Here's how the part is built. I have some questions about the finished solid (model axes, mm). A direction names the side the tool comes from. Round coordinates to 2 decimals unless told otherwise and drop trailing zeros. Order: outer loops, then holes, each group sorted by start corner. A loop starts at its lowest first (then second) coordinate and runs counter-clockwise, first axis right, second up. Notation, with made-up numbers: (60.25, 30.5) -> (117.25, 30.5) arc R22 cw to (117.25, 60.5) -> close; hole circle Ø6 at (63.25, -15.5). An arc over 180 degrees is marked (long way). Answer in a Markdown table with one row per item.
```python
from build123d import *

# Parameters (mm, degrees)
F1_DEPTH = 82
F2_R     = 5.5
F3_DEPTH = 16.001
F4_R     = 14
F5_R     = 14


with BuildPart() as f1:
    # F0 (on Front) → F1 (new body)
    with BuildSketch(Plane.XZ):
        with BuildLine():
            Line((0, 16), (0, 0))
            Line((0, 0), (38, 0))
            Line((38, 0), (38, -4))
            Line((38, -4), (98, -4))
            Line((98, -4), (98, 0))
            Line((98, 0), (136, 0))
            Line((136, 0), (136, 16))
            Line((136, 16), (92, 16))
            ThreePointArc((92, 16), (90.070466, 13.197483), (86.763932, 14))
            Line((86.763932, 14), (49.236068, 14))
            ThreePointArc((49.236068, 14), (45.929534, 13.197483), (44, 16))
            Line((44, 16), (0, 16))
        make_face()
    extrude(amount=-F1_DEPTH)

    # F2 (on Top) → F3 (cut, through all)
    with BuildSketch(Plane.XY):
        with Locations((14, 68)):
            Circle(F2_R)
        with Locations((14, 14)):
            Circle(F2_R)
        with Locations((122, 68)):
            Circle(F2_R)
        with Locations((122, 14)):
            Circle(F2_R)
    extrude(amount=F3_DEPTH, mode=Mode.SUBTRACT)

    # F4
    f4_edges = [f1.edges().sort_by_distance(p)[0] for p in [
        (136, 0, 8),
        (136, 82, 8),
    ]]
    fillet(f4_edges, radius=F4_R)

    # F5
    f5_edges = [f1.edges().sort_by_distance(p)[0] for p in [
        (0, 0, 8),
        (0, 82, 8),
    ]]
    fillet(f5_edges, radius=F5_R)


solid = f1.part
```
1. For pin 1 Ø19 at (x, y) = (69, 23.5) entering from +Z; pin 2 Ø14.5 at (x, y) = (122, 68) entering from -Z; pin 3 Ø4.5 at (y, z) = (22, -2.5) entering from -X, each with a flat end and sliding along its axis, tell me the tip position at first contact or that it passes through.
Numbers:
| item | result |
|---|---|
| pin 1 | stops at z = 14 |
| pin 2 | stops at z = 0 |
| pin 3 | stops at x = 38 |
2. For faces 1 (the face through (98, 40, -2)), 2 (the face through (38, 40, -2)), 3 (the face through (19.08, 11.89, 7.89)), 4 (the face through (68, 40, 14)), which set-ups out of +Z, -Z, +X, -X, +Y, -Y let a thin tool reach every point of the face, with its end or its side?
Numbers:
| item | result |
|---|---|
| face 1 | -Z, +X, +Y, -Y |
| face 2 | -Z, -X, +Y, -Y |
| face 3 | +Z, -Z |
| face 4 | +Z, +Y, -Y |
3. We'd pull the mould along X, two halves only. Please class faces 5 (the face through (4, 77.8, 7.9)), 6 (the face through (131.8, 78, 8.1)), 7 (the face through (13.284, 73.453, 7.888)): released by +X, released by -X, zero draft, split by the parting line, or undercut.
Numbers:
| item | result |
|---|---|
| face 5 | released by -X |
| face 6 | released by +X |
| face 7 | undercut |
4. Suppose I cut it at D-D on x = 66. Write out the boundary of the cut face in (y, z), then the cut area to 3 significant figures.
Numbers:
| item | result |
|---|---|
| outline | (0, -4) -> (82, -4) -> (82, 14) -> (0, 14) -> close |
| area | 1,480 mm2 |
5. Suppose I cut it at C-C on x = 10. Write out the boundary of the cut face in (y, z).
Numbers:
| item | result |
|---|---|
| outline | (0.58, 0) -> (10.23, 0) -> (10.23, 16) -> (0.58, 16) -> close; (17.77, 0) -> (64.23, 0) -> (64.23, 16) -> (17.77, 16) -> close; (71.77, 0) -> (81.42, 0) -> (81.42, 16) -> (71.77, 16) -> close |
6. Please list where these lines run through material, in increasing order: line 1 along Y through (x, z) = (122, 10.75); line 2 along X through (y, z) = (14, 7.75); line 3 along Y through (x, z) = (127, 0.5).
Numbers:
| item | result |
|---|---|
| line 1 | y = 0 to 8.5, 19.5 to 62.5, 73.5 to 82 |
| line 2 | x = 0 to 8.5, 19.5 to 116.5, 127.5 to 136 |
| line 3 | y = 0.92 to 11.71, 16.29 to 65.71, 70.29 to 81.08 |
7. Suppose I cut it at A-A on y = 47. Write out the boundary of the cut face in (x, z), then the cut area to 3 significant figures.
Numbers:
| item | result |
|---|---|
| outline | (0, 0) -> (38, 0) -> (38, -4) -> (98, -4) -> (98, 0) -> (136, 0) -> (136, 16) -> (92, 16) arc R3 cw to (86.76, 14) -> (49.24, 14) arc R3 cw to (44, 16) -> (0, 16) -> close |
| area | 2,310 mm2 |
8. Suppose I cut it at B-B on z = 3.75. Write out the boundary of the cut face in (x, y), then the cut area to 3 significant figures.
Numbers:
| item | result |
|---|---|
| outline | (0, 14) arc R14 ccw to (14, 0) -> (122, 0) arc R14 ccw to (136, 14) -> (136, 68) arc R14 ccw to (122, 82) -> (14, 82) arc R14 ccw to (0, 68) -> close; hole circle Ø11 at (14, 14); hole circle Ø11 at (14, 68); hole circle Ø11 at (122, 14); hole circle Ø11 at (122, 68) |
| area | 10,600 mm2 |
